Autodesk Fusion 360 part; units mm, degrees
sketch "Sketch1" plane through (0, 0, 0) normal (0, 1, 0) x (1, 0, 0)
  line L0 (0, 0) -> (19, 0)
  line L1 (19, 0) -> (19, 22.5)
  line L2 (19, 22.5) -> (0, 22.5)
  line L3 (0, 22.5) -> (0, 0)
  dimension "d1" = 19
  dimension "d2" = 22.5
extrude "Extrude1" add sketch "Sketch1" along normal blind 20 makes body 1
sketch "Sketch2" plane through (0, 0, 0) normal (0, 0, 1) x (1, 0, 0)
  line L0 (0, 0) -> (19, 0)
  line L1 (19, 0) -> (19, 20)
  line L2 (19, 20) -> (0, 20)
  line L3 (0, 20) -> (0, 0)
  line L4 (20.6, 7.5) -> (-1.6, 7.5)
  line L5 (-1.6, 7.5) -> (-1.6, 0)
  line L6 (-1.6, 0) -> (20.6, 0)
  line L7 (20.6, 0) -> (20.6, 7.5)
  line L8 (19, 7.5) -> (19, 0)
  line L9 (0, 7.5) -> (0, 0)
  dimension "d5" = 1.6
  dimension "d6" = 1.6
  dimension "d7" = 7.5
extrude "Extrude2" add sketch "Sketch2" against normal blind 22.25 separate body contours L3 L4 L5 L6 L9 | L1 L4 L6 L7 L8 makes body 2 at (19, 2.5, -7.4167) makes body 3 at (-1.6, 5, -7.4167)
extrude "Extrude3" add sketch "Sketch2" along normal blind 1.6 separate body contours L0 L1 L3 L4 L6 L8 L9 | L3 L4 L5 L6 L9 | L1 L4 L6 L7 L8 makes body 4
combine "Combine1" operation add target body 2 tool bodies 4 3
sketch "Sketch3" plane through (0, 0, -22.25) normal (0, 0, -1) x (-1, 0, 0)
  line L0 (1.6, 0) -> (1.6, 7.5)
  line L1 (1.6, 7.5) -> (0, 7.5)
  line L2 (0, 7.5) -> (0, 0)
  line L3 (0, 0) -> (1.6, 0)
  line L4 (1.6, 0) -> (20.1, 0)
  line L5 (20.1, 0) -> (20.1, 7.5)
  line L6 (20.1, 7.5) -> (1.6, 7.5)
  line L7 (1.6, 7.5) -> (1.6, 0)
  line L8 (-20.6, 0) -> (-28.1, 0)
  line L9 (-28.1, 0) -> (-28.1, 7.5)
  line L10 (-28.1, 7.5) -> (-20.6, 7.5)
  line L11 (-20.6, 7.5) -> (-20.6, 0)
  line L12 (-19, 7.5) -> (-20.6, 7.5)
  circle A0 centre (-24.35, 3.75) radius 1.75
  circle A1 centre (16.35, 3.75) radius 1.75
  point P0 (-20.6, 0)
  dimension "d13" = 7.5
  dimension "d16" = 3.5
  dimension "d17" = 3.75
  dimension "d18" = 3.75
  dimension "d19" = 3.75
  dimension "d20" = 3.75
  dimension "d29" = 40.7
extrude "Extrude4" add sketch "Sketch3" against normal blind 1.6 contours L0 L4 L5 L6 L7 | L8 L9 L10 L11 bodies 2
chamfer "Chamfer1" distance 11.5 angle 45 1 edges at (-1.6, 3.75, -20.65) on bodies 2
sketch "Sketch6" plane through (0, 7.5, 0) normal (0, 1, 0) x (-1, 0, 0)
  line L0 (-28.1, -22.25) -> (-19, -22.25)
  line L1 (-19, -22.25) -> (-19, 0)
  line L2 (-19, 0) -> (0, 0)
  line L3 (0, 0) -> (0, -22.25)
  line L4 (0, -22.25) -> (20.1, -22.25)
  line L5 (20.1, -22.25) -> (20.1, -20.65)
  line L6 (20.1, -20.65) -> (13.1, -20.65)
  line L7 (13.1, -20.65) -> (1.6, -9.15)
  line L8 (1.6, -9.15) -> (1.6, 1.6)
  line L9 (1.6, 1.6) -> (-20.6, 1.6)
  line L10 (-20.6, 1.6) -> (-20.6, -20.65)
  line L11 (-20.6, -20.65) -> (-28.1, -20.65)
  line L12 (-28.1, -20.65) -> (-28.1, -22.25)
  line L13 (1.6, -11.4127) -> (10.8373, -20.65)
  line L14 (10.8373, -20.65) -> (1.6, -20.65)
  line L15 (1.6, -20.65) -> (1.6, -11.4127)
  dimension "d23" = 1.6
  dimension "d24" = 1.6
  dimension "d25" = 1.6
extrude "Extrude5" cut sketch "Sketch6" against normal blind 11 contours L13 L14 L15 bodies 2
hidden bodies 1
equation "d17 = ( 7.5 / 2 ) * 1 mm"
equation "d18 = ( 7.5 / 2 ) * 1 mm"
equation "d19 = ( 7.5 / 2 ) * 1 mm"
equation "d20 = ( 7.5 / 2 ) * 1 mm"
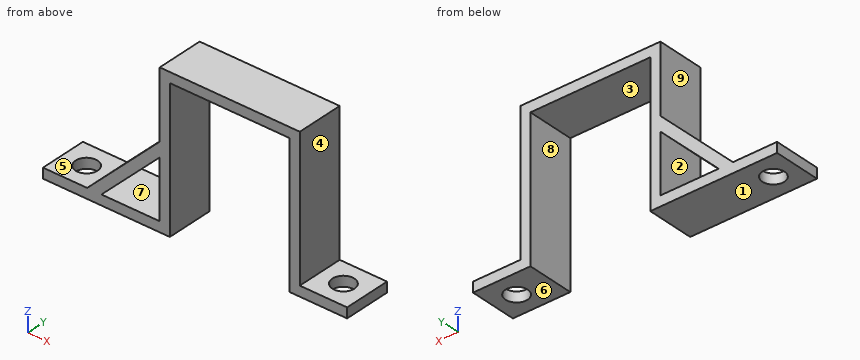
The model under review builds one solid part; all positions refer to its coordinate system, in mm. Face numbers are marked on the shaded views. A direction names the side the tool comes from. Round coordinates to 2 decimals unless told otherwise and drop trailing zeros. Write each loop counter-clockwise with the first axis right and the second up, starting at its lowest first coordinate (ties: lowest second). Pieces come first, ordered by that corner, then holes. Notation, with made-up numbers: (13.25, 84.25) - (24.25, 84.25) arc R28 ccw to (24.25, 115.25) - close; hole circle Ø5 at (73.5, 32). An arc over 180 degrees is marked (long way). One line per item, written item: value. Start each with the question number.
1. Consider section D-D on x = 17.5. Write out the cut boundary in (y, z).
2. Machinability: for the marked faces 1, 2, 3, 4 and 5, which of the approach directions +Z, -Z, +X, -X, +Y, -Y give a long, thin tool a straight path to every point of the face, cutting with its end or side? Answer none if there is none.
3. Consider section C-C on z = -20. Write out the cut boundary in (x, y), and give its area (3 significant figures).
4. Clearance check with flat-ended pins moving along their axes: P1, Ø3.5, axis at x = -17, y = 5.5, coming from the +Z side; P2, Ø4, axis at x = -4.5, y = 3.5, coming from the +Z side; P3, Ø4, axis at y = 3, z = -6, coming from the -X side. State where each tip first meets the part, or that it passes through.
5. Consider section A-A on z = -1.75. Write out the cut boundary in (x, y), and give its area (3 significant figures).
6. Consider section B-B on x = -16.35. Write out the cut boundary in (y, z), and give its area (3 significant figures).
7. The part is to be moulded in two halves that separate along X. For the marked faces 6, 7, 8 and 9, say which applies: released by +X, released by -X, zero draft, split by the parting line, or undercut.
8. To check wall thickness, follow L1, parallel to Y at x = -16.35, z = -21.4; L2, parallel to X at y = 4.75, z = -2.5; L3, parallel to X at y = 2.5, z = -20.25. State the ranges of each line that lie inside material, in increasing order. Write a range as from..to.
Checks:
1. outline: (0, 0) - (7.5, 0) - (7.5, 1.6) - (0, 1.6) - close
2. face 1: -Z, +X, -X, +Y, -Y
2. face 2: +Y, -Y
2. face 3: -Z, +Y, -Y
2. face 4: +Z, +X, +Y, -Y
2. face 5: +Z, -X, +Y, -Y
3. outline: (-12.45, 0) - (-10.19, 0) - (-10.19, 7.5) - (-12.45, 7.5) - close; (-1.6, 0) - (0, 0) - (0, 7.5) - (-1.6, 7.5) - close; (19, 0) - (20.6, 0) - (20.6, 7.5) - (19, 7.5) - close
3. area: 41.0 mm^2
4. P1: stops at z = -20.65
4. P2: stops at z = -10.05
4. P3: stops at x = -1.6
5. outline: (-1.6, 0) - (0, 0) - (0, 7.5) - (-1.6, 7.5) - close; (19, 0) - (20.6, 0) - (20.6, 7.5) - (19, 7.5) - close
5. area: 24.0 mm^2
6. outline: (0, -22.25) - (2, -22.25) - (2, -20.65) - (0, -20.65) - close; (5.5, -22.25) - (7.5, -22.25) - (7.5, -20.65) - (5.5, -20.65) - close
6. area: 6.40 mm^2
7. face 6: zero draft
7. face 7: undercut
7. face 8: undercut
7. face 9: released by -X
8. L1: y = 0..2, 5.5..7.5
8. L2: x = -1.6..0, 19..20.6
8. L3: x = -12.7..-10.44, -1.6..0, 19..20.6
